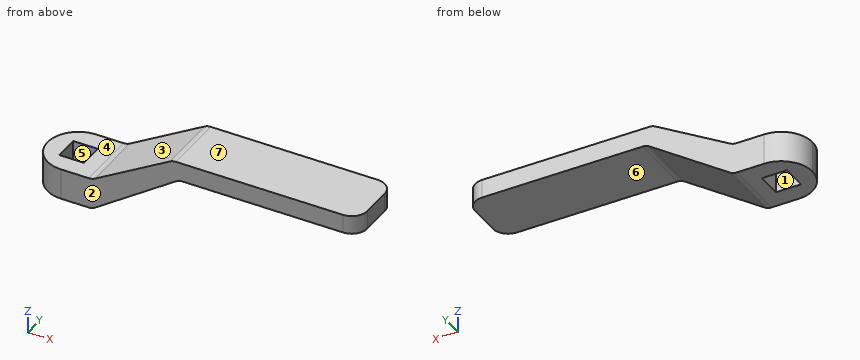
```python
from build123d import *

# Parameters (mm, degrees)
F1_DEPTH = 10
F2_W     = 8
F2_H     = 8
F3_DEPTH = 10
F4_R     = 9.99999
F5_R     = 4
F6_R     = 5


# Not quite as in the source:
# - a fillet or chamfer is up to 0.001 mm smaller than in the source, because OpenCascade refuses the exact size


with BuildPart() as f1:
    # F0 (on Front) → F1 (new body, symmetric)
    with BuildSketch(Plane.XZ):
        Polygon((35.9807621135, 20), (10, 5), (-10, 5), (-10, -5), (10, -5), (37.9807621135, 14), (95.9807621135, 14), (95.9807621135, 20), align=None)
    extrude(amount=F1_DEPTH, both=True)

    # F2 (on face) → F3 (cut, through all)
    with BuildSketch(Plane.XY.offset(5)):
        Rectangle(F2_W, F2_H)
    extrude(amount=-F3_DEPTH, mode=Mode.SUBTRACT)

    # F4 (radius 10 in the source; OpenCascade refuses exactly that, so slightly less here)
    f4_edges = [f1.edges().sort_by_distance(p)[0] for p in [
        (-10, -10, 0),
        (-10, 10, 0),
    ]]
    fillet(f4_edges, radius=F4_R)

    # F5
    f5_edges = [f1.edges().sort_by_distance(p)[0] for p in [
        (35.980762, 0, 20),
        (10, 0, 5),
        (10, 0, -5),
        (37.980762, 0, 14),
    ]]
    fillet(f5_edges, radius=F5_R)

    # F6
    f6_edges = [f1.edges().sort_by_distance(p)[0] for p in [
        (95.980762, 10, 17),
        (95.980762, -10, 17),
    ]]
    fillet(f6_edges, radius=F6_R)


solid = f1.part
```
Read the model definition and answer for the solid it produces. Units are mm, in the model's axes. Face numbers are marked on the shaded views. A direction names the side the tool comes from. Coordinates: 2 decimals unless noted, no trailing zeros. Write each loop counter-clockwise with the first axis right and the second up, starting at its lowest first coordinate (ties: lowest second). Pieces come first, ordered by that corner, then holes. Notation, with made-up numbers: (-2.75, -19) - (30.25, -19) arc R24 ccw to (30.25, 13) - close; hole circle Ø8 at (39, 29.5). An arc over 180 degrees is marked (long way). Answer as a JSON object with one key per item and string values. Group by question number.
1. Consider L1, parallel to Z at x = 88, y = 0; L2, parallel to X at y = 1, z = -4; L3, parallel to X at y = -3, z = 2.5. Determine where each line is inside the solid, lowest interval first. Write a range as [from, to].
2. A cutting plane is placed at C-C (x = 48). Determine the outline of the cut face in (y, z).
3. A cutting plane is placed at A-A (y = 1.5). Determine the outline of the cut face in (x, z).
4. Which of the six approach directions +Z, -Z, +X, -X, +Y, -Y give full straight-line access (tool end or side, diameter ignored) to the marked faces 4, 5, 6 and 7?
5. The mould has two halves that part along Y. Classify the marked faces 1, 2 and 3: +Y half, -Y half, draft (parallel to the pull), parting line (faces both ways), or undercut.
6. Each of these flat-tipped pins is pushed along its axis until it touches: P1, Ø10, axis at y = -4, z = 14.5, coming from the -X side; P2, Ø6, axis at x = 18, y = 1, coming from the +Z side; P3, Ø9.5, axis at x = 3.5, y = -3, coming from the +Z side. Where does it stop, or does it pass through?
7. A cutting plane is placed at D-D (z = 15). Determine the outline of the cut face in (x, y), plus the area to 3 significant figures.
Worked out:
{
 "1": {"L1": "z = [14, 20]", "L2": "x = [-9.95, -4], [4, 11.47]", "L3": "x = [-9.54, -4], [4, 21.05]"},
 "2": {"outline": "(-10, 14) - (10, 14) - (10, 20) - (-10, 20) - close"},
 "3": {"outline": "(-9.89, -5) - (-4, -5) - (-4, 5) - (-9.89, 5) - close; (4, -5) - (8.77, -5) arc R4 ccw to (11.02, -4.31) - (36.96, 13.31) arc R4 cw to (39.21, 14) - (95.98, 14) - (95.98, 20) - (37.05, 20) arc R4 ccw to (35.05, 19.46) - (10.93, 5.54) arc R4 cw to (8.93, 5) - (4, 5) - close"},
 "4": {"face 4": "+Z, -X, +Y, -Y", "face 5": "+Z, -Z", "face 6": "-Z, +X, +Y, -Y", "face 7": "+Z, +X, -X, +Y, -Y"},
 "5": {"face 1": "undercut", "face 2": "-Y half", "face 3": "draft"},
 "6": {"P1": "stops at x = 17.79", "P2": "stops at z = 11.35", "P3": "stops at z = 5"},
 "7": {"outline": "(27.32, -10) - (90.98, -10) arc R5 ccw to (95.98, -5) - (95.98, 5) arc R5 ccw to (90.98, 10) - (27.32, 10) - close", "area": "1,360 mm²"}
}
